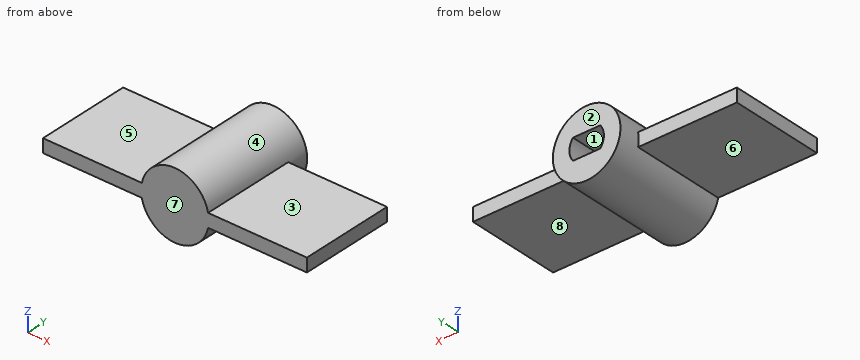
```python
from build123d import *

# Parameters (mm, degrees)
SKETCH_W     = 39
SKETCH_H     = 14
PAD_DEPTH    = 2
SKETCH001_R  = 5
PAD001_DEPTH = 17.199
POCKET_DEPTH = 8


with BuildPart() as part:
    # Sketch → Pad (new body)
    with BuildSketch(Plane.XY):
        with Locations((19.5, 7)):
            Rectangle(SKETCH_W, SKETCH_H)
    extrude(amount=PAD_DEPTH)

    # Sketch001 (on Face1 of Pad) → Pad001 (join)
    with BuildSketch(Plane.XZ):
        with Locations((19.5, 1)):
            Circle(SKETCH001_R)
    extrude(amount=-PAD001_DEPTH)

    # Sketch002 (on Face14 of Pad001) → Pocket (cut)
    with BuildSketch(Plane(origin=(0, 17.199, 0), x_dir=(-1, 0, 0), z_dir=(0, 1, 0))):
        with BuildLine():
            ThreePointArc((-21.524846, 2.55), (-22.05, 1), (-21.524846, -0.55))
            Line((-17.475154, -0.55), (-21.524846, -0.55))
            ThreePointArc((-17.475154, -0.55), (-16.95, 1), (-17.475154, 2.55))
            Line((-21.524846, 2.55), (-17.475154, 2.55))
        make_face()
    extrude(amount=-POCKET_DEPTH, mode=Mode.SUBTRACT)


solid = part.part
```
Could you check a few things on this model? Use its own coordinates, in mm. Face numbers are marked on the shaded views. A direction names the side the tool comes from. Give positions to 0.01 mm unless a question says otherwise; leave off trailing zeros. Write each loop counter-clockwise with the first axis right and the second up, starting at its lowest first coordinate (ties: lowest second). Pieces come first, ordered by that corner, then holes. Notation, with made-up numbers: (10, 62.5) - (17, 62.5) arc R17 ccw to (17, 88.5) - close; hole circle Ø1 at (61, -2.5). An arc over 180 degrees is marked (long way). One line per item, written item: value. Start each with the question number.
Item 1: Please list where these lines run through material, in increasing order: line 1 (Z direction, x = 33, y = 2.75); line 2 (Y direction, x = 5, z = 1); line 3 (X direction, y = 14, z = 2.25). Write a range as from..to.
Item 2: Imagine slicing it at C-C, the plane y = 7.25. List the corners of the cut face in (x, z) for me.
Item 3: Imagine slicing it at D-D, the plane x = 19.5. List the corners of the cut face in (y, z) for me.
Item 4: Which directions (+Z, -Z, +X, -X, +Y, -Y) give clear straight access to the entire face, cutting with the end or side of a thin tool? Please do the marked faces 5, 6, 7 and 8.
Item 5: I'm going to push flat-ended pins straight in: pin 1 (1.5 mm diameter, centred on x = 14, z = -2, fed in from -Y); pin 2 (6 mm diameter, centred on x = 5, y = 3, fed in from -Z); pin 3 (0.6 mm diameter, centred on x = 29.5, z = 1, fed in from +Y); pin 4 (4 mm diameter, centred on x = 5, y = 7, fed in from +Z). Where does each tip first touch, or does it pass through?
Item 6: Imagine slicing it at A-A, the plane y = 11.25. List the corners of the cut face in (x, z) for me.
Item 7: Imagine slicing it at B-B, the plane z = 1. List the corners of the cut face in (x, y) for me, and give its area (3 significant figures).
Item 8: If we mould it in two halves opening along Z, with no side actions, what happens to the marked faces 1, 2, 3 and 4? For each: +Z half, -Z half, draft (parallel to the pull), parting line (faces both ways), or undercut.
Geometry says:
1. line 1: 0..2
1. line 2: 0..14
1. line 3: 14.66..17.28, 21.72..24.34
2. outline: (0, 0) - (14.6, 0) arc R5 ccw to (24.4, 0) - (39, 0) - (39, 2) - (24.4, 2) arc R5 ccw to (14.6, 2) - (0, 2) - close
3. outline: (0, -4) - (17.2, -4) - (17.2, -0.55) - (9.2, -0.55) - (9.2, 2.55) - (17.2, 2.55) - (17.2, 6) - (0, 6) - close
4. face 5: +Z, -X, +Y, -Y
4. face 6: -Z, -X, +Y, -Y
4. face 7: +Z, -Z, +X, -X, -Y
4. face 8: -Z, +X, +Y, -Y
5. pin 1: through
5. pin 2: z = 0
5. pin 3: y = 14
5. pin 4: z = 2
6. outline: (0, 0) - (14.6, 0) arc R5 ccw to (24.4, 0) - (39, 0) - (39, 2) - (24.4, 2) arc R5 ccw to (14.6, 2) - (0, 2) - close; hole (17.48, -0.55) - (21.52, -0.55) arc R2.55 ccw to (21.52, 2.55) - (17.48, 2.55) arc R2.55 ccw to start
7. outline: (0, 0) - (39, 0) - (39, 14) - (24.5, 14) - (24.5, 17.2) - (22.05, 17.2) - (22.05, 9.2) - (16.95, 9.2) - (16.95, 17.2) - (14.5, 17.2) - (14.5, 14) - (0, 14) - close
7. area: 537 mm^2
8. face 1: undercut
8. face 2: draft
8. face 3: +Z half
8. face 4: parting line
